```python
from build123d import *

# Parameters (mm, degrees)
F0_W     = 11
F0_H     = 30
F1_DEPTH = 24
F3_DEPTH = 11
F4_R     = 5
F4_R_2   = 2.5
F5_DEPTH = 41.001


with BuildPart() as f1:
    # F0 (on Right) → F1 (new body, symmetric)
    with BuildSketch(Plane.YZ):
        with BuildLine():
            Line((-56, 0), (-30, 0))
            ThreePointArc((-30, 0), (-29.4730143031, 5.5983415304), (-27.9105714739, 11))
            Line((-27.9105714739, 11), (-56, 11))
            Line((-56, 11), (-56, 0))
        make_face()
        with BuildLine():
            ThreePointArc((-27.9105714739, 11), (-29.4730143031, 5.5983415304), (-30, 0))
            Line((-30, 0), (-19, 0))
            ThreePointArc((-19, 0), (-18.1017503893, 5.7729223833), (-15.4919333848, 11))
            Line((-15.4919333848, 11), (-27.9105714739, 11))
        make_face()
        with BuildLine():
            Line((15.4919333848, 11), (27.9105714739, 11))
            ThreePointArc((27.9105714739, 11), (0, 30), (-27.9105714739, 11))
            Line((-27.9105714739, 11), (-15.4919333848, 11))
            ThreePointArc((-15.4919333848, 11), (0, 19), (15.4919333848, 11))
        make_face()
        with BuildLine():
            Line((19, 0), (30, 0))
            ThreePointArc((30, 0), (29.4730143031, 5.5983415304), (27.9105714739, 11))
            Line((27.9105714739, 11), (15.4919333848, 11))
            ThreePointArc((15.4919333848, 11), (18.1017503893, 5.7729223833), (19, 0))
        make_face()
        with BuildLine():
            ThreePointArc((27.9105714739, 11), (29.4730143031, 5.5983415304), (30, 0))
            Line((30, 0), (51, 0))
            Line((51, 0), (51, 11))
            Line((51, 11), (40, 11))
            Line((40, 11), (27.9105714739, 11))
        make_face()
        with Locations((45.5, 26)):
            Rectangle(F0_W, F0_H)
    extrude(amount=F1_DEPTH, both=True)

    # F2 (on face) → F3 (cut, through all)
    with BuildSketch(Plane(origin=(0, 51, 0), x_dir=(-1, 0, 0), z_dir=(0, 1, 0))):
        with BuildLine():
            Line((-6.5220605694, 25.4945768912), (-6.5220605694, 24.5054231088))
            ThreePointArc((-6.5220605694, 24.5054231088), (-0.2061620785, 18.4624639527), (6.4779394306, 24.0954663604))
            Line((6.4779394306, 24.0954663604), (6.4779394306, 25.9045336396))
            ThreePointArc((6.4779394306, 25.9045336396), (-0.2061620785, 31.5375360473), (-6.5220605694, 25.4945768912))
        make_face()
        with BuildLine():
            Line((-6.5220605694, 41), (-6.5220605694, 25.4945768912))
            ThreePointArc((-6.5220605694, 25.4945768912), (-0.2061620785, 31.5375360473), (6.4779394306, 25.9045336396))
            Line((6.4779394306, 25.9045336396), (6.4779394306, 41))
            Line((6.4779394306, 41), (-6.5220605694, 41))
        make_face()
    extrude(amount=-F3_DEPTH, mode=Mode.SUBTRACT)

    # F4 (on Top) → F5 (cut, through all)
    with BuildSketch(Plane.XY):
        with Locations((11, -42.3406362534)):
            Circle(F4_R)
        with Locations((-11, -42.3406362534)):
            Circle(F4_R)
        Circle(F4_R_2)
    extrude(amount=F5_DEPTH, mode=Mode.SUBTRACT)


solid = f1.part
```
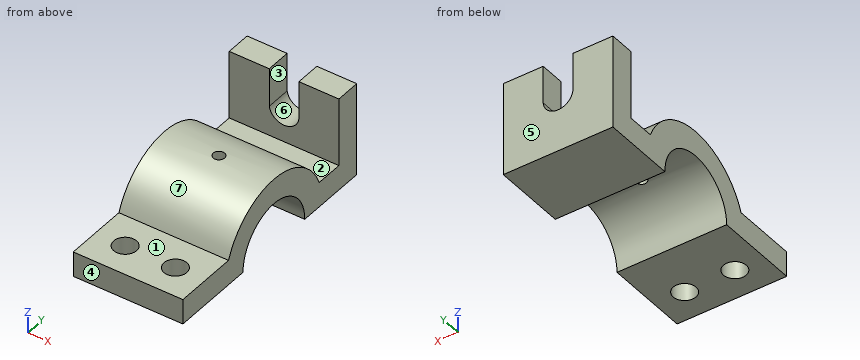
Read the model definition and answer for the solid it produces. Units are mm, in the model's axes. Face numbers are marked on the shaded views. A direction names the side the tool comes from. Coordinates: 2 decimals unless noted, no trailing zeros. Write each loop counter-clockwise with the first axis right and the second up, starting at its lowest first coordinate (ties: lowest second). Pieces come first, ordered by that corner, then holes. Notation, with made-up numbers: (-28, -13) - (7, -13) arc R30 cw to (7, 10) - close; hole circle Ø6 at (66.5, -12). An arc over 180 degrees is marked (long way). Answer as a JSON object with one key per item and string values. Group by question number.
1. Consider L1, parallel to Y at x = -11, z = 6; L2, parallel to Y at x = 11, z = 7.5; L3, parallel to Y at x = 18.5, z = 33. Determine where each line is inside the solid, lowest interval first. Write a range as [from, to].
2. A cutting plane is placed at A-A (z = 3). Determine the outline of the cut face in (x, y), plus the area to 3 significant figures.
3. A cutting plane is placed at B-B (x = -11). Determine the outline of the cut face in (y, z), plus the area to 3 significant figures.
4. Which of the six approach directions +Z, -Z, +X, -X, +Y, -Y give full straight-line access (tool end or side, diameter ignored) to the marked faces 1, 2 and 3?
5. A cutting plane is placed at D-D (z = 32.5). Determine the outline of the cut face in (x, y).
6. The mould has two halves that part along Y. Classify the marked faces 4, 5, 6 and 7: +Y half, -Y half, draft (parallel to the pull), parting line (faces both ways), or undercut.
7. Each of these flat-tipped pins is pushed along its axis until it touches: P1, Ø9, axis at x = -2.5, z = 31, coming from the -Y side; P2, Ø11.5, axis at x = 11, y = -42.34, coming from the +Z side; P3, Ø4, axis at x = -7, z = 34, coming from the -Y side. Where does it stop, or does it pass through?
8. A cutting plane is placed at C-C (y = 41). Determine the outline of the cut face in (x, z), plus the area to 3 significant figures.
Worked out:
{
 "1": {"L1": "y = [-56, -47.34], [-37.34, -18.03], [18.03, 51]", "L2": "y = [-56, -47.34], [-37.34, -17.46], [17.46, 51]", "L3": "y = [40, 51]"},
 "2": {"outline": "(-24, -56) - (24, -56) - (24, -18.76) - (-24, -18.76) - close; (-24, 18.76) - (24, 18.76) - (24, 51) - (-24, 51) - close; hole circle Ø10 at (-11, -42.34); hole circle Ø10 at (11, -42.34)", "area": "3,180 mm²"},
 "3": {"outline": "(-56, 0) - (-47.34, 0) - (-47.34, 11) - (-56, 11) - close; (-37.34, 0) - (-19, 0) arc R19 cw to (19, 0) - (51, 0) - (51, 41) - (40, 41) - (40, 11) - (27.91, 11) arc R30 ccw to (-27.91, 11) - (-37.34, 11) - close", "area": "1,600 mm²"},
 "4": {"face 1": "+Z, +X, -X, -Y", "face 2": "+Z, +X, -X", "face 3": "+Z, +Y"},
 "5": {"outline": "(-24, 40) - (-6.48, 40) - (-6.48, 51) - (-24, 51) - close; (6.52, 40) - (24, 40) - (24, 51) - (6.52, 51) - close"},
 "6": {"face 4": "-Y half", "face 5": "+Y half", "face 6": "draft", "face 7": "undercut"},
 "7": {"P1": "stops at y = -14.06", "P2": "stops at z = 11", "P3": "stops at y = 40"},
 "8": {"outline": "(-24, 0) - (24, 0) - (24, 41) - (6.52, 41) - (6.52, 24.51) arc R6.54 cw to (-6.48, 24.1) - (-6.48, 41) - (-24, 41) - close", "area": "1,690 mm²"}
}
